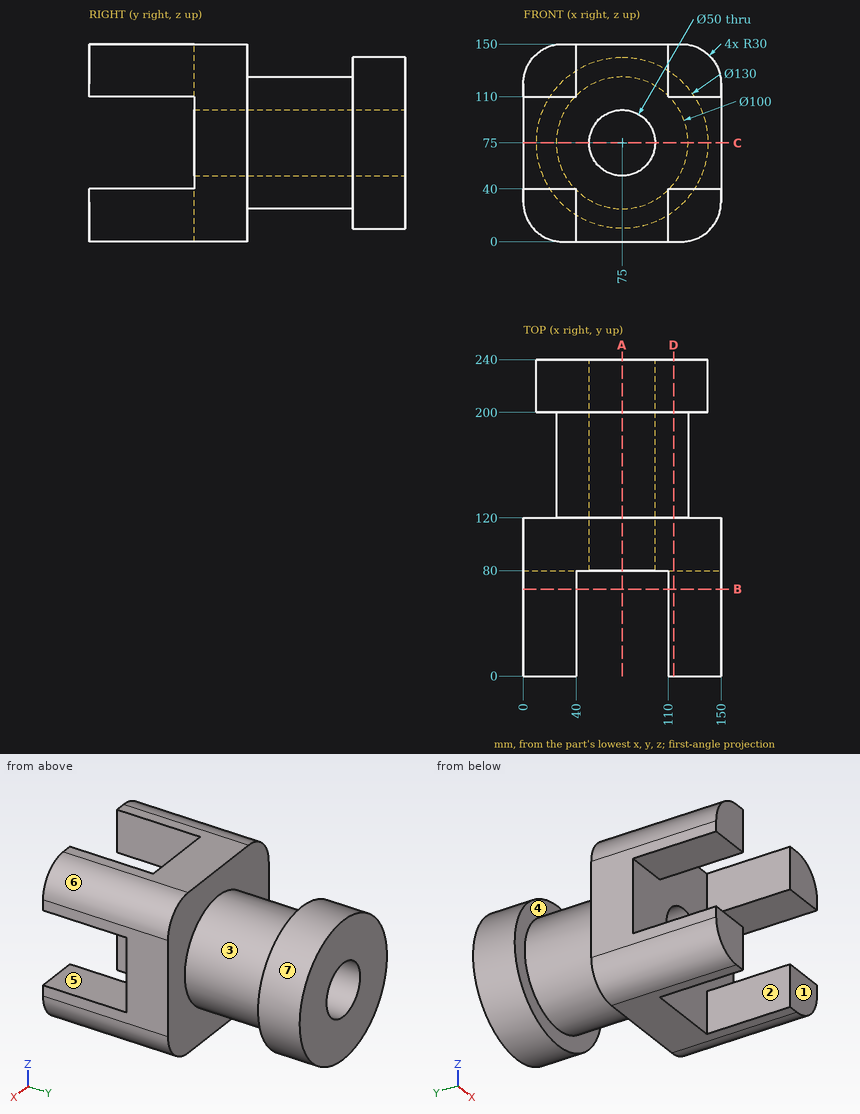
Design review of the part shown in the three views and the two pictorial views. Dimensions are in mm from the part's minimum x, y and z. A direction names the side the tool comes from. Coordinates: 2 decimals unless noted, no trailing zeros. Order: outer loops, then holes, each group sorted by start corner. A loop starts at its lowest first (then second) coordinate and runs counter-clockwise, first axis right, second up. Notation, with made-up numbers: (-1, 16) -> (28, 16) arc R9 cw to (28, 32) -> close; hole circle Ø7 at (68, 24). An arc over 180 degrees is marked (long way). Use one line per item in the form item = value. Start each with the question number.
(1) For the marked faces 4, 5, 6 and 7, list the 3-axis set-ups (+Z, -Z, +X, -X, +Y, -Y) from which the entire face can be reached by the end or side of a thin tool; tool diameter is ignored.
(2) Insertion check: pin 1 (3 mm diameter, centred on y = 205, z = 105.5, fed in from -X); pin 2 (12 mm diameter, centred on x = 131.5, y = 48.5, fed in from -Z); pin 3 (3 mm diameter, centred on x = 78.5, z = 43.5, fed in from -Y); pin 4 (10 mm diameter, centred on x = 43, y = 64.5, fed in from +Z). Each pin has a flat end and moves straight along its axis. Give the tip position at first contact, or say it passes through.
(3) The part is to be moulded in two halves that separate along X. For the marked faces 1, 2 and 3, say which applies: +X half, -X half, draft (parallel to the pull), parting line (faces both ways), or undercut.
(4) Add section C-C on z = 75. State the section outline as (x, y) points.
(5) For probe 1 along X at (y, z) = (190, 75); probe 2 along Y at (x, z) = (65, 30.5); probe 3 along Y at (x, z) = (76, 137.5), list the stretches that pass through material, from the lowest coordinate up.
(6) Add section D-D on x = 114. State the section outline as (y, z) points, plus the area to 3 significant figures.
(7) Add section B-B on y = 66. State the section outline as (x, z) points.
(8) Add section A-A on x = 75. State the section outline as (y, z) points.
Answer block:
q1.face_4 = none
q1.face_5 = +X, -X, -Y
q1.face_6 = +Z, +X, +Y, -Y
q1.face_7 = +Y
q2.pin_1 = 16.83
q2.pin_2 = 0.51
q2.pin_3 = 80
q2.pin_4 = 150
q3.face_1 = draft
q3.face_2 = undercut
q3.face_3 = parting line
q4.outline = (0, 80) -> (50, 80) -> (50, 240) -> (10, 240) -> (10, 200) -> (25, 200) -> (25, 120) -> (0, 120) -> close; (100, 80) -> (150, 80) -> (150, 120) -> (125, 120) -> (125, 200) -> (140, 200) -> (140, 240) -> (100, 240) -> close
q5.probe_1 = 25 to 50, 100 to 125
q5.probe_2 = 80 to 240
q5.probe_3 = 80 to 120, 200 to 240
q6.outline = (0, 0) -> (120, 0) -> (120, 43.71) -> (200, 43.71) -> (200, 23) -> (240, 23) -> (240, 127) -> (200, 127) -> (200, 106.29) -> (120, 106.29) -> (120, 150) -> (0, 150) -> (0, 110) -> (80, 110) -> (80, 40) -> (0, 40) -> close
q6.area = 21,600 mm²
q7.outline = (0, 30) arc R30 ccw to (30, 0) -> (40, 0) -> (40, 40) -> (0, 40) -> close; (0, 110) -> (40, 110) -> (40, 150) -> (30, 150) arc R30 ccw to (0, 120) -> close; (110, 0) -> (120, 0) arc R30 ccw to (150, 30) -> (150, 40) -> (110, 40) -> close; (110, 110) -> (150, 110) -> (150, 120) arc R30 ccw to (120, 150) -> (110, 150) -> close
q8.outline = (80, 0) -> (120, 0) -> (120, 25) -> (200, 25) -> (200, 10) -> (240, 10) -> (240, 50) -> (80, 50) -> close; (80, 100) -> (240, 100) -> (240, 140) -> (200, 140) -> (200, 125) -> (120, 125) -> (120, 150) -> (80, 150) -> close
